Part print with two shaded views. Sizes in mm from the minimum x, y, z corner. Give positions to 0.01 mm unless a question says otherwise; leave off trailing zeros. Write each loop counter-clockwise with the first axis right and the second up, starting at its lowest first coordinate (ties: lowest second). Pieces come first, ordered by that corner, then holes. Notation, with made-up numbers: (-24.75, 7.5) -> (16.25, 7.5) arc R22 cw to (16.25, 35.5) -> close; hole circle Ø10 at (-27.75, 39). An arc over 180 degrees is marked (long way). Write item = value, one per line. Start each with the question number.
Q1. Wall check: line 1 (X direction, y = 6, z = 4.1); line 2 (X direction, y = 4.5, z = 2.2) (1 decimal); line 3 (X direction, y = 4.25, z = 0.5) (1 decimal). Give the ranges that are in metal, low to high.
Q2. Saw through at A-A, the plane z = 1.1. List the corners of the cut face in (x, y).
Q3. Drop a flat-ended pin along its axis: P1, Ø2, axis at x = 75.5, y = 3, coming from the +Z side. Give the stop position or say it passes through.
Q4. Saw through at C-C, the plane y = 5. Give the number of separate pieces and of enclosed holes in the cut face.
Q5. Saw through at B-B, the plane x = 44.5. List the corners of the cut face in (y, z).
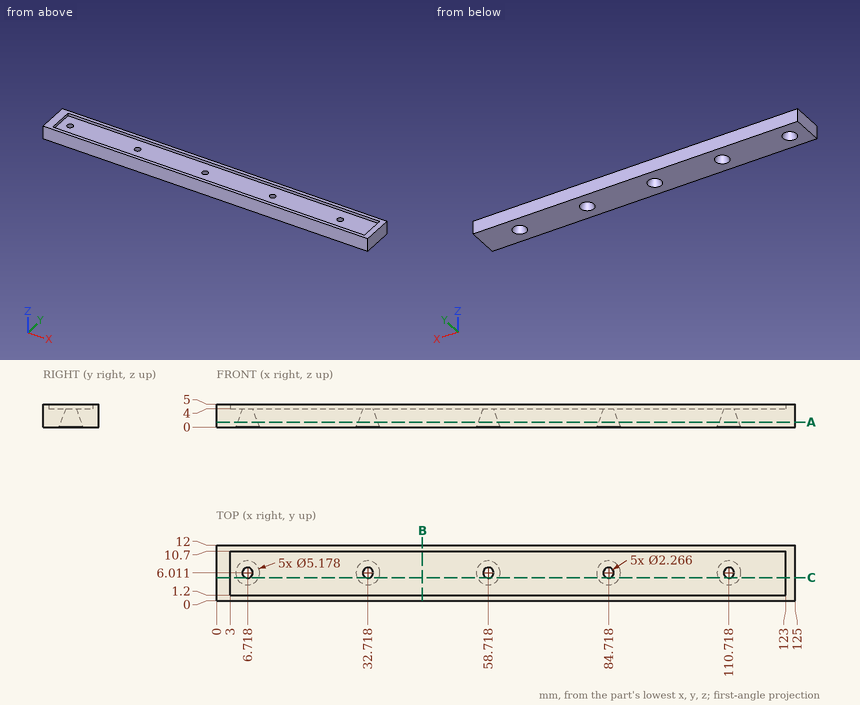
Report:
q1.line_1 = 0 to 3, 123 to 125
q1.line_2 = 0 to 5.8, 7.7 to 31.8, 33.7 to 57.8, 59.7 to 83.8, 85.7 to 109.8, 111.7 to 125
q1.line_3 = 0 to 5.1, 8.4 to 31.1, 34.4 to 57.1, 60.4 to 83.1, 86.4 to 109.1, 112.4 to 125
q2.outline = (0, 0) -> (125, 0) -> (125, 12) -> (0, 12) -> close; hole circle Ø4.38 at (6.72, 6.01); hole circle Ø4.38 at (32.72, 6.01); hole circle Ø4.38 at (58.72, 6.01); hole circle Ø4.38 at (84.72, 6.01); hole circle Ø4.38 at (110.72, 6.01)
q3.P1 = 4
q4.separate_pieces = 6
q4.enclosed_holes = 0
q5.outline = (0, 0) -> (12, 0) -> (12, 5) -> (10.7, 5) -> (10.7, 4) -> (1.2, 4) -> (1.2, 5) -> (0, 5) -> close
